```python
from build123d import *

# Parameters (mm, degrees)
F0_R     = 2
F1_DEPTH = 25


with BuildPart() as f1:
    # F0 (on Top) → F1 (new body)
    with BuildSketch(Plane.XY):
        with BuildLine():
            Line((-5.59017, 50), (-12.928932, 50))
            ThreePointArc((-12.928932, 50), (-14.842349, 49.619398), (-16.464466, 48.535534))
            Line((-16.464466, 48.535534), (-48.535534, 16.464466))
            ThreePointArc((-48.535534, 16.464466), (-49.619398, 14.842349), (-50, 12.928932))
            Line((-50, 12.928932), (-50, 5.59017))
            ThreePointArc((-50, 5.59017), (-49.253254, 2.961514), (-47.236068, 1.118034))
            Line((-47.236068, 1.118034), (-45, 0))
            Line((-45, 0), (-47.236068, -1.118034))
            ThreePointArc((-47.236068, -1.118034), (-49.253254, -2.961514), (-50, -5.59017))
            Line((-50, -5.59017), (-50, -12.928932))
            ThreePointArc((-50, -12.928932), (-49.619398, -14.842349), (-48.535534, -16.464466))
            Line((-48.535534, -16.464466), (-16.464466, -48.535534))
            ThreePointArc((-16.464466, -48.535534), (-14.842349, -49.619398), (-12.928932, -50))
            Line((-12.928932, -50), (-5.59017, -50))
            ThreePointArc((-5.59017, -50), (-2.961514, -49.253254), (-1.118034, -47.236068))
            Line((-1.118034, -47.236068), (0, -45))
            Line((0, -45), (1.118034, -47.236068))
            ThreePointArc((1.118034, -47.236068), (2.961514, -49.253254), (5.59017, -50))
            Line((5.59017, -50), (12.928932, -50))
            ThreePointArc((12.928932, -50), (14.842349, -49.619398), (16.464466, -48.535534))
            Line((16.464466, -48.535534), (48.535534, -16.464466))
            ThreePointArc((48.535534, -16.464466), (49.619398, -14.842349), (50, -12.928932))
            Line((50, -12.928932), (50, -5.59017))
            ThreePointArc((50, -5.59017), (49.253254, -2.961514), (47.236068, -1.118034))
            Line((47.236068, -1.118034), (45, 0))
            Line((45, 0), (47.236068, 1.118034))
            ThreePointArc((47.236068, 1.118034), (49.253254, 2.961514), (50, 5.59017))
            Line((50, 5.59017), (50, 12.928932))
            ThreePointArc((50, 12.928932), (49.619398, 14.842349), (48.535534, 16.464466))
            Line((48.535534, 16.464466), (16.464466, 48.535534))
            ThreePointArc((16.464466, 48.535534), (14.842349, 49.619398), (12.928932, 50))
            Line((12.928932, 50), (5.59017, 50))
            ThreePointArc((5.59017, 50), (2.961514, 49.253254), (1.118034, 47.236068))
            Line((1.118034, 47.236068), (0, 45))
            Line((0, 45), (-1.118034, 47.236068))
            ThreePointArc((-1.118034, 47.236068), (-2.961514, 49.253254), (-5.59017, 50))
        make_face()
        with Locations((-22.923625, -31.551663)):
            Circle(F0_R, mode=Mode.SUBTRACT)
        with Locations((-12.051663, -37.091204)):
            Circle(F0_R, mode=Mode.SUBTRACT)
        with Locations((-11.863186, -28.640266)):
            Circle(F0_R, mode=Mode.SUBTRACT)
        with Locations((-31.551663, -22.923625)):
            Circle(F0_R, mode=Mode.SUBTRACT)
        with Locations((-37.091204, -12.051663)):
            Circle(F0_R, mode=Mode.SUBTRACT)
        with Locations((-28.640266, -11.863186)):
            Circle(F0_R, mode=Mode.SUBTRACT)
        with Locations((-21.92031, -21.92031)):
            Circle(F0_R, mode=Mode.SUBTRACT)
        with Locations((-11.5, -19.918584)):
            Circle(F0_R, mode=Mode.SUBTRACT)
        with Locations((-19.918584, -11.5)):
            Circle(F0_R, mode=Mode.SUBTRACT)
        with Locations((0, -39)):
            Circle(F0_R, mode=Mode.SUBTRACT)
        with Locations((12.051663, -37.091204)):
            Circle(F0_R, mode=Mode.SUBTRACT)
        with Locations((0, -31)):
            Circle(F0_R, mode=Mode.SUBTRACT)
        with Locations((11.863186, -28.640266)):
            Circle(F0_R, mode=Mode.SUBTRACT)
        with Locations((22.923625, -31.551663)):
            Circle(F0_R, mode=Mode.SUBTRACT)
        with Locations((0, -23)):
            Circle(F0_R, mode=Mode.SUBTRACT)
        with Locations((11.5, -19.918584)):
            Circle(F0_R, mode=Mode.SUBTRACT)
        with Locations((21.92031, -21.92031)):
            Circle(F0_R, mode=Mode.SUBTRACT)
        with Locations((19.918584, -11.5)):
            Circle(F0_R, mode=Mode.SUBTRACT)
        with Locations((31.551663, -22.923625)):
            Circle(F0_R, mode=Mode.SUBTRACT)
        with Locations((28.640266, -11.863186)):
            Circle(F0_R, mode=Mode.SUBTRACT)
        with Locations((37.091204, -12.051663)):
            Circle(F0_R, mode=Mode.SUBTRACT)
        with Locations((-39, 0)):
            Circle(F0_R, mode=Mode.SUBTRACT)
        with Locations((-31, 0)):
            Circle(F0_R, mode=Mode.SUBTRACT)
        with Locations((-37.091204, 12.051663)):
            Circle(F0_R, mode=Mode.SUBTRACT)
        with Locations((-28.640266, 11.863186)):
            Circle(F0_R, mode=Mode.SUBTRACT)
        with Locations((-31.551663, 22.923625)):
            Circle(F0_R, mode=Mode.SUBTRACT)
        with Locations((-23, 0)):
            Circle(F0_R, mode=Mode.SUBTRACT)
        with Locations((-19.918584, 11.5)):
            Circle(F0_R, mode=Mode.SUBTRACT)
        with Locations((-21.92031, 21.92031)):
            Circle(F0_R, mode=Mode.SUBTRACT)
        with Locations((-11.5, 19.918584)):
            Circle(F0_R, mode=Mode.SUBTRACT)
        with Locations((-22.923625, 31.551663)):
            Circle(F0_R, mode=Mode.SUBTRACT)
        with Locations((-11.863186, 28.640266)):
            Circle(F0_R, mode=Mode.SUBTRACT)
        with Locations((-12.051663, 37.091204)):
            Circle(F0_R, mode=Mode.SUBTRACT)
        with BuildLine():
            ThreePointArc((-12.247449, 2.5), (-8.838835, 8.838835), (-2.5, 12.247449))
            Line((-2.5, 12.247449), (0, 17.5))
            Line((0, 17.5), (2.5, 12.247449))
            ThreePointArc((2.5, 12.247449), (8.838835, 8.838835), (12.247449, 2.5))
            Line((12.247449, 2.5), (17.5, 0))
            Line((17.5, 0), (12.247449, -2.5))
            ThreePointArc((12.247449, -2.5), (8.838835, -8.838835), (2.5, -12.247449))
            Line((2.5, -12.247449), (0, -17.5))
            Line((0, -17.5), (-2.5, -12.247449))
            ThreePointArc((-2.5, -12.247449), (-8.838835, -8.838835), (-12.247449, -2.5))
            Line((-12.247449, -2.5), (-17.5, 0))
            Line((-17.5, 0), (-12.247449, 2.5))
        make_face(mode=Mode.SUBTRACT)
        with Locations((23, 0)):
            Circle(F0_R, mode=Mode.SUBTRACT)
        with Locations((19.918584, 11.5)):
            Circle(F0_R, mode=Mode.SUBTRACT)
        with Locations((0, 23)):
            Circle(F0_R, mode=Mode.SUBTRACT)
        with Locations((11.5, 19.918584)):
            Circle(F0_R, mode=Mode.SUBTRACT)
        with Locations((21.92031, 21.92031)):
            Circle(F0_R, mode=Mode.SUBTRACT)
        with Locations((31, 0)):
            Circle(F0_R, mode=Mode.SUBTRACT)
        with Locations((28.640266, 11.863186)):
            Circle(F0_R, mode=Mode.SUBTRACT)
        with Locations((37.091204, 12.051663)):
            Circle(F0_R, mode=Mode.SUBTRACT)
        with Locations((39, 0)):
            Circle(F0_R, mode=Mode.SUBTRACT)
        with Locations((31.551663, 22.923625)):
            Circle(F0_R, mode=Mode.SUBTRACT)
        with Locations((0, 31)):
            Circle(F0_R, mode=Mode.SUBTRACT)
        with Locations((11.863186, 28.640266)):
            Circle(F0_R, mode=Mode.SUBTRACT)
        with Locations((12.051663, 37.091204)):
            Circle(F0_R, mode=Mode.SUBTRACT)
        with Locations((22.923625, 31.551663)):
            Circle(F0_R, mode=Mode.SUBTRACT)
        with Locations((0, 39)):
            Circle(F0_R, mode=Mode.SUBTRACT)
    extrude(amount=F1_DEPTH)


solid = f1.part
```
Input: part model. Units: mm. Frame: model coordinates. Round coordinates to 2 decimals unless told otherwise and drop trailing zeros. Loops run counter-clockwise (first coordinate to the right, second up) from the corner with the lowest first, then second, coordinate; pieces in that order, holes last. Notation, with made-up numbers: M 89.5,68 L 125.5,68 A27 ccw 125.5,85 Z; hole C 62.5,64.5 d8. An arc over 180 degrees is marked long. Answer in a Markdown table with one row per item. Add a question column.
1. Section B-B (z = 7). Give the number of separate pieces and of enclosed holes in the cut face, and give its area (3 significant figures).
2. Mould query, pull axis X, two halves, no side actions, for faces 1 (the face through (18.445, -10.148, 12.325)), 2 (the face through (-49.27, 2.99, 12.32)), 3 (the face through (9, -50, 12)). Classes: released by +X, released by -X, zero draft, split by the parting line, or undercut.
3. Ray query, probe 1 along Y at (x, z) = (23.5, 13); probe 2 along X at (y, z) = (32, 10); probe 3 along X at (y, z) = (38.5, 17). Return the intervals inside material, ascending.
4. Contact query for flat-ended pins moving along their axis: pin 1 (3 mm diameter, centred on x = -26.5, z = 11.5, fed in from +Y); pin 2 (3 mm diameter, centred on x = 24.5, y = -22, fed in from -Z); pin 3 (6 mm diameter, centred on y = -35, z = 7.5, fed in from -X); pin 4 (10 mm diameter, centred on y = 35, z = 17, fed in from +X). Output: stop coordinate, or through.
5. Section A-A (y = -42.5). Output: boundary loops of the cut face in (x, z).
Values follow:
| question | item | result |
|---|---|---|
| 1 | separate pieces | 1 |
| 1 | enclosed holes | 49 |
| 1 | area | 6,340 mm^2 |
| 2 | face 1 | undercut |
| 2 | face 2 | released by -X |
| 2 | face 3 | zero draft |
| 3 | probe 1 | -41.5 to -33.47, -29.64 to -23.15, -20.69 to -1.94, 1.94 to 20.69, 23.15 to 29.64, 33.47 to 41.5 |
| 3 | probe 2 | -33 to -24.87, -20.97 to -1.73, 1.73 to 20.97, 24.87 to 33 |
| 3 | probe 3 | -26.5 to -13.47, -10.63 to -1.94, 1.94 to 10.63, 13.47 to 26.5 |
| 4 | pin 1 | y = 40 |
| 4 | pin 2 | z = 0 |
| 4 | pin 3 | x = -33 |
| 4 | pin 4 | x = 35 |
| 5 | outline | M -22.5,0 L 22.5,0 L 22.5,25 L -22.5,25 Z |
